```python
from build123d import *

# Parameters (mm, degrees)
F0_R     = 17
F0_R_2   = 10
F1_DEPTH = 26


with BuildPart() as f1:
    # F0 (on Front) → F1 (new body)
    with BuildSketch(Plane.XZ):
        with BuildLine():
            Line((-73.556583, 102.53989), (-27.834874, -11.190164))
            ThreePointArc((-27.834874, -11.190164), (14.80033, -26.095023), (23.88951, 18.146385))
            Line((23.88951, 18.146385), (-0.699871, 58.827717))
            Line((-0.699871, 58.827717), (-37.883752, 120.345727))
            ThreePointArc((-37.883752, 120.345727), (-52.886286, 129.887992), (-69.559346, 123.712237))
            ThreePointArc((-69.559346, 123.712237), (-74.652818, 113.710357), (-73.556583, 102.53989))
        make_face()
        Circle(F0_R, mode=Mode.SUBTRACT)
        with Locations((-55, 110)):
            Circle(F0_R_2, mode=Mode.SUBTRACT)
        with BuildLine():
            Line((-37.883752, 120.345727), (-0.699871, 58.827717))
            ThreePointArc((-0.699871, 58.827717), (-1.208181, 74.474703), (11.879405, 83.06549))
            ThreePointArc((11.879405, 83.06549), (35.878556, 102.299329), (26.299489, 131.525024))
            ThreePointArc((26.299489, 131.525024), (-23.184125, 146.687816), (-69.559346, 123.712237))
            ThreePointArc((-69.559346, 123.712237), (-52.886286, 129.887992), (-37.883752, 120.345727))
        make_face()
        with Locations((10, 110)):
            Circle(F0_R_2, mode=Mode.SUBTRACT)
    extrude(amount=F1_DEPTH)


solid = f1.part
```
The model under review builds one solid part; all positions refer to its coordinate system, in mm. A direction names the side the tool comes from. Round coordinates to 2 decimals unless told otherwise and drop trailing zeros. Write each loop counter-clockwise with the first axis right and the second up, starting at its lowest first coordinate (ties: lowest second). Pieces come first, ordered by that corner, then holes. Notation, with made-up numbers: M 64.25,-9.5 L 88.25,-9.5 A21 ccw 88.25,16.5 Z; hole C 31,86.25 d6. An arc over 180 degrees is marked long. Use CSV: the item, a comma, the result in double quotes. Start each with the question number.
(1) We need section D-D, the plane z = 10. State the section outline as (x, y) points.
(2) We need section C-C, the plane y = -22. State the section outline as (x, z) points, then the cut area to 3 significant figures.
(3) For line 1 along Z through (x, y) = (17.5, -22); line 2 along Z through (x, y) = (10, -5.25); line 3 along X through (y, z) = (-23.5, 113.5), list the stretches that pass through material, from the lowest coordinate up.
(4) We need section B-B, the plane x = -55. State the section outline as (y, z) points.
(5) We need section A-A, the plane z = 110. State the section outline as (x, y) points.
(6) The part is to be moulded in two halves that separate along Z. For faces 1 (the face through (-51.016, -12.818, 46.471)), 2 (the face through (-56.302, -12.818, 119.915)), 3 (the face through (-22.444, -12.818, 146.744)), 4 (the face through (-74.62, -12.82, 113.87)), say which applies: +Z half, -Z half, draft (parallel to the pull), parting line (faces both ways), or undercut.
(7) Clearance check with flat-ended pins moving along their axes: P1, Ø5, axis at y = -22.5, z = 61, coming from the +X side; P2, Ø1, axis at x = -3, y = -23, coming from the -Z side; P3, Ø6, axis at y = -15, z = 103.5, coming from the +X side; P4, Ø23, axis at x = -55, z = 110, coming from the +Y side. State where each tip first meets the part, or that it passes through.
(8) Tool access review of faces 5 (the face through (14.173, -12.818, -26.441)), 6 (the face through (11.77, -12.82, 38.2)): name each direction out of +Z, -Z, +X, -X, +Y, -Y from which nothing blocks a thin tool from reaching the whole face with its end or side.
Findings:
1,outline,"M -36.35,-26 L -13.75,-26 L -13.75,0 L -36.35,0 Z; M 13.75,-26 L 28.28,-26 L 28.28,0 L 13.75,0 Z"
2,outline,"M -73.56,102.54 L -27.83,-11.19 A30 ccw long 23.89,18.15 L -0.7,58.83 A16 cw 11.88,83.07 A27 ccw 26.3,131.53 A70 ccw -69.56,123.71 A20 ccw Z; hole C -55,110 d20; hole C 0,0 d34; hole C 10,110 d20"
2,area,"10,800 mm^2"
3,line 1,"-24.37 to 28.72, 84.06 to 103.39, 116.61 to 137.54"
3,line 2,"-28.28 to -13.75, 13.75 to 41.13, 82.82 to 100, 120 to 141.29"
3,line 3,"-74.69 to -64.37, -45.63 to 0.63, 19.37 to 36.77"
4,outline,"M -26,56.38 L 0,56.38 L 0,100 L -26,100 Z; M -26,120 L 0,120 L 0,136.03 L -26,136.03 Z"
5,outline,"M -75,-26 L -65,-26 L -65,0 L -75,0 Z; M -45,-26 L 0,-26 L 0,0 L -45,0 Z; M 20,-26 L 37,-26 L 37,0 L 20,0 Z"
6,face 1,"-Z half"
6,face 2,"undercut"
6,face 3,"+Z half"
6,face 4,"parting line"
7,P1,"x = -0.5"
7,P2,"z = -29.9"
7,P3,"x = 36.77"
7,P4,"y = 0"
8,face 5,"+Y, -Y"
8,face 6,"+X, +Y, -Y"
